from build123d import *

# Parameters (mm, degrees)
EXTRUDE_1_DEPTH             = 3
HOLE_WIZARD_M3_1_AT_2_COUNT = 2
HOLE_WIZARD_M3_1_AT_2_PITCH = 89
HOLE_WIZARD_M3_1_AT_3_COUNT = 2
HOLE_WIZARD_M3_1_AT_3_PITCH = 139.767316539
HOLE_WIZARD_M3_1_AT_4_COUNT = 2
HOLE_WIZARD_M3_1_AT_4_PITCH = 158.615198724
HOLE_WIZARD_M3_1_AT_5_COUNT = 2
HOLE_WIZARD_M3_1_AT_5_PITCH = 105.5
FILLET_1_R                  = 3
FILLET_2_R                  = 3
CUT_EXTRUDE_1_DEPTH         = 1.2
SKETCH_5_W                  = 15
SKETCH_5_H                  = 88
CUT_EXTRUDE_2_DEPTH         = 0.8
FILLET_5_R                  = 3
FILLET_6_R                  = 5
FILLET_7_R                  = 3
SKETCH_6_W                  = 1
SKETCH_6_H                  = 16
SKETCH_6_H_2                = 12
SKETCH_6_W_2                = 12
SKETCH_6_H_3                = 1
EXTRUDE_2_DEPTH             = 1
FILLET_8_R                  = 3
CHAMFER_1_SIZE              = 1
EXTRUDE_4_DEPTH             = 1.2
CUT_EXTRUDE_3_DEPTH         = 10
CUT_EXTRUDE_5_DEPTH         = 1.5
CUT_EXTRUDE_6_DEPTH         = 0.4
FILLET_9_R                  = 2
FILLET_10_R                 = 4


with BuildPart() as part:
    # 草图1 → 凸台-拉伸1 (new body)
    with BuildSketch(Plane.XY):
        Polygon((15, 96), (15, 72), (0, 72), (0, 10), (20, 0), (145, 0), (145, 96), align=None)
    extrude(amount=EXTRUDE_1_DEPTH)

    # 草图2 → M3 平头机械螺钉的锥形沉头孔1 (revolve, cut)
    with BuildSketch(Plane(origin=(141.5, 92.5, 3), x_dir=(0, -1, 0), z_dir=(1, 0, 0))):
        Polygon((0, 0), (0, 3), (1.7, 3), (1.7, 1.45), (3.15, 0), align=None)
    hole_wizard_m3_1 = revolve(axis=Axis((141.5, 92.5, 9.35), (0, 0, -1)), mode=Mode.SUBTRACT)

    # M3 平头机械螺钉的锥形沉头孔1 at 2: M3 平头机械螺钉的锥形沉头孔1 ×2
    with Locations(*[(0, -i * HOLE_WIZARD_M3_1_AT_2_PITCH, 0) for i in range(1, HOLE_WIZARD_M3_1_AT_2_COUNT)]):
        add(hole_wizard_m3_1, mode=Mode.SUBTRACT)

    # M3 平头机械螺钉的锥形沉头孔1 at 3: M3 平头机械螺钉的锥形沉头孔1 ×2
    with Locations(*[Vector(-0.9837779203696774, -0.1793906446644101, 0) * (i * HOLE_WIZARD_M3_1_AT_3_PITCH) for i in range(1, HOLE_WIZARD_M3_1_AT_3_COUNT)]):
        add(hole_wizard_m3_1, mode=Mode.SUBTRACT)

    # M3 平头机械螺钉的锥形沉头孔1 at 4: M3 平头机械螺钉的锥形沉头孔1 ×2
    with Locations(*[Vector(-0.8668778345720617, -0.4985206313961874, 0) * (i * HOLE_WIZARD_M3_1_AT_4_PITCH) for i in range(1, HOLE_WIZARD_M3_1_AT_4_COUNT)]):
        add(hole_wizard_m3_1, mode=Mode.SUBTRACT)

    # M3 平头机械螺钉的锥形沉头孔1 at 5: M3 平头机械螺钉的锥形沉头孔1 ×2
    with Locations(*[(-i * HOLE_WIZARD_M3_1_AT_5_PITCH, 0, 0) for i in range(1, HOLE_WIZARD_M3_1_AT_5_COUNT)]):
        add(hole_wizard_m3_1, mode=Mode.SUBTRACT)

    # 圆角1
    fillet_1_edges = [part.edges().sort_by_distance(p)[0] for p in [
        (145, 0, 1.5),
        (145, 96, 1.5),
    ]]
    fillet(fillet_1_edges, radius=FILLET_1_R)

    # 圆角2
    fillet_2_edges = [part.edges().sort_by_distance(p)[0] for p in [
        (20, 0, 1.5),
        (0, 10, 1.5),
        (0, 72, 1.5),
        (15, 96, 1.5),
    ]]
    fillet(fillet_2_edges, radius=FILLET_2_R)

    # 草图4 → 切除-拉伸1 (cut)
    with BuildSketch(Plane(origin=(0, 0, 0), x_dir=(-1, 0, 0), z_dir=(0, 0, -1))):
        Polygon((-133.585786438, 92), (-141, 84.585786438), (-141, 12.121320344), (-132.878679656, 4), (-22.062305899, 4), (-13, 8.531152949), (-13, 24), (-4, 27), (-4, 50.47410222), (-19.5, 68.946282906), (-19.5, 91), (-27.171572875, 91), (-32.171572875, 86), (-39.828427125, 86), (-45.828427125, 92), align=None)
    extrude(amount=-CUT_EXTRUDE_1_DEPTH, mode=Mode.SUBTRACT)

    # 草图5 → 切除-拉伸2 (cut)
    with BuildSketch(Plane(origin=(0, 0, 1.2), x_dir=(-1, 0, 0), z_dir=(0, 0, -1))):
        with Locations((-85.5, 48)):
            Rectangle(SKETCH_5_W, SKETCH_5_H)
    extrude(amount=-CUT_EXTRUDE_2_DEPTH, mode=Mode.SUBTRACT)

    # 圆角5
    fillet_5_edges = [part.edges().sort_by_distance(p)[0] for p in [
        (13, 8.531152949, 0.6),
        (22.062305899, 4, 0.6),
        (132.878679656, 4, 0.6),
        (141, 12.121320344, 0.6),
        (141, 84.585786438, 0.6),
        (133.585786438, 92, 0.6),
        (4, 50.47410222, 0.6),
        (4, 27, 0.6),
        (45.828427125, 92, 0.6),
        (27.171572875, 91, 0.6),
        (19.5, 91, 0.6),
    ]]
    fillet(fillet_5_edges, radius=FILLET_5_R)

    # 圆角6
    fillet_6_edges = [part.edges().sort_by_distance(p)[0] for p in [
        (39.828427125, 86, 0.6),
        (32.171572875, 86, 0.6),
        (19.5, 68.946282906, 0.6),
        (13, 24, 0.6),
    ]]
    fillet(fillet_6_edges, radius=FILLET_6_R)

    # 圆角7
    fillet_7_edges = [part.edges().sort_by_distance(p)[0] for p in [
        (78, 4, 1.6),
        (93, 4, 1.6),
        (78, 92, 1.6),
        (93, 92, 1.6),
    ]]
    fillet(fillet_7_edges, radius=FILLET_7_R)

    # 草图6 → 凸台-拉伸2 (add)
    with BuildSketch(Plane(origin=(0, 0, 0), x_dir=(-1, 0, 0), z_dir=(0, 0, -1))):
        with Locations((-141.5, 48)):
            Rectangle(SKETCH_6_W, SKETCH_6_H)
        with Locations((-3.5, 40)):
            Rectangle(SKETCH_6_W, SKETCH_6_H_2)
        with Locations((-76, 3.5)):
            Rectangle(SKETCH_6_W_2, SKETCH_6_H_3)
        with Locations((-76, 92.5)):
            Rectangle(SKETCH_6_W_2, SKETCH_6_H_3)
    extrude(amount=EXTRUDE_2_DEPTH)

    # 圆角8
    fillet_8_edges = [part.edges().sort_by_distance(p)[0] for p in [
        (15, 72, 1.5),
    ]]
    fillet(fillet_8_edges, radius=FILLET_8_R)

    # 倒角1
    chamfer_1_edges = [part.edges().sort_by_distance(p)[0] for p in [
        (3.5, 46, -1),
        (3.5, 34, -1),
        (70, 3.5, -1),
        (82, 3.5, -1),
        (141.5, 56, -1),
        (141.5, 40, -1),
        (82, 92.5, -1),
        (70, 92.5, -1),
    ]]
    chamfer(chamfer_1_edges, length=CHAMFER_1_SIZE - 0.0001)  # a hair under: the kernel refuses the full size

    # 草图9 → 凸台-拉伸4 (add)
    with BuildSketch(Plane(origin=(0, 0, 1.2), x_dir=(-1, 0, 0), z_dir=(0, 0, -1))):
        with BuildLine():
            Line((-95, 92), (-95, 34))
            Line((-95, 34), (-141, 34))
            Line((-141, 34), (-141, 83.343145751))
            ThreePointArc((-141, 83.343145751), (-140.771638598, 84.491196048), (-140.121320344, 85.464466094))
            Line((-140.121320344, 85.464466094), (-134.464466094, 91.121320344))
            ThreePointArc((-134.464466094, 91.121320344), (-133.491196048, 91.771638598), (-132.343145751, 92))
            Line((-132.343145751, 92), (-95, 92))
        make_face()
    extrude(amount=EXTRUDE_4_DEPTH)

    # 草图7 → 切除-拉伸3 (cut)
    with BuildSketch(Plane.XY.offset(3)):
        with BuildLine():
            Line((100, 86), (134, 86))
            ThreePointArc((134, 86), (134.707106781, 85.707106781), (135, 85))
            Line((135, 85), (135, 42))
            ThreePointArc((135, 42), (134.707106781, 41.292893219), (134, 41))
            Line((134, 41), (100, 41))
            ThreePointArc((100, 41), (99.292893219, 41.292893219), (99, 42))
            Line((99, 42), (99, 85))
            ThreePointArc((99, 85), (99.292893219, 85.707106781), (100, 86))
        make_face()
    extrude(amount=-CUT_EXTRUDE_3_DEPTH, mode=Mode.SUBTRACT)

    # 草图10 → 切除-拉伸5 (cut)
    with BuildSketch(Plane(origin=(0, 0, 0), x_dir=(-1, 0, 0), z_dir=(0, 0, -1))):
        with BuildLine():
            Line((-135, 89), (-99, 89))
            ThreePointArc((-99, 89), (-96.878679656, 88.121320344), (-96, 86))
            Line((-96, 86), (-96, 41))
            ThreePointArc((-96, 41), (-96.878679656, 38.878679656), (-99, 38))
            Line((-99, 38), (-135, 38))
            ThreePointArc((-135, 38), (-137.121320344, 38.878679656), (-138, 41))
            Line((-138, 41), (-138, 86))
            ThreePointArc((-138, 86), (-137.121320344, 88.121320344), (-135, 89))
        make_face()
    extrude(amount=-CUT_EXTRUDE_5_DEPTH, mode=Mode.SUBTRACT)

    # 草图12 → 切除-拉伸6 (cut)
    with BuildSketch(Plane(origin=(0, 0, 1.5), x_dir=(-1, 0, 0), z_dir=(0, 0, -1))):
        with BuildLine():
            Line((-135, 38), (-99, 38))
            ThreePointArc((-99, 38), (-96.878679656, 38.878679656), (-96, 41))
            Line((-96, 41), (-96, 86))
            ThreePointArc((-96, 86), (-96.878679656, 88.121320344), (-99, 89))
            Line((-99, 89), (-135, 89))
            ThreePointArc((-135, 89), (-137.121320344, 88.121320344), (-138, 86))
            Line((-138, 86), (-138, 41))
            ThreePointArc((-138, 41), (-137.121320344, 38.878679656), (-135, 38))
        make_face()
        with BuildLine():
            Line((-135, 39.5), (-99, 39.5))
            ThreePointArc((-99, 39.5), (-97.939339828, 39.939339828), (-97.5, 41))
            Line((-97.5, 41), (-97.5, 86))
            ThreePointArc((-97.5, 86), (-97.939339828, 87.060660172), (-99, 87.5))
            Line((-99, 87.5), (-135, 87.5))
            ThreePointArc((-135, 87.5), (-136.060660172, 87.060660172), (-136.5, 86))
            Line((-136.5, 86), (-136.5, 41))
            ThreePointArc((-136.5, 41), (-136.060660172, 39.939339828), (-135, 39.5))
        make_face(mode=Mode.SUBTRACT)
    extrude(amount=-CUT_EXTRUDE_6_DEPTH, mode=Mode.SUBTRACT)

    # 圆角9
    fillet_9_edges = [part.edges().sort_by_distance(p)[0] for p in [
        (141, 34, 0.6),
        (95, 92, 0.6),
    ]]
    fillet(fillet_9_edges, radius=FILLET_9_R)

    # 圆角10
    fillet_10_edges = [part.edges().sort_by_distance(p)[0] for p in [
        (95, 34, 0.6),
    ]]
    fillet(fillet_10_edges, radius=FILLET_10_R)


solid = part.part
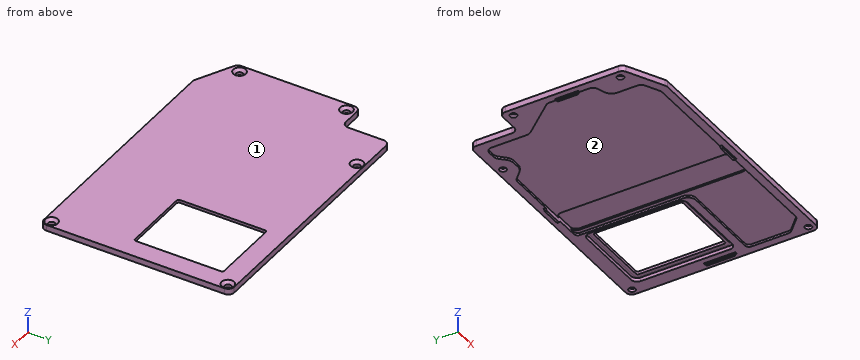
Part model, mm, in its own coordinate system. Face numbers are marked on the shaded views. Coordinates: 2 decimals unless noted, no trailing zeros. Order: outer loops, then holes, each group sorted by start corner. A loop starts at its lowest first (then second) coordinate and runs counter-clockwise, first axis right, second up. Notation, with made-up numbers: M 5,-17 L 32,-17 A31 cw 32,13 Z; hole C -18,84 d3. An arc over 180 degrees is marked long. Use a Markdown table: item, result.
(1) Cut at C-C on x = 103. Write the cut outline in (y, z).
A:
| item | result |
|---|---|
| outline | M 0,0 L 4,0 L 4,1.2 L 34,1.2 L 34,0 L 38,0 L 38,1.9 L 39.5,1.9 L 39.5,1.5 L 41,1.5 L 41,3 L 0,3 Z; M 86,1.5 L 87.5,1.5 L 87.5,1.9 L 89,1.9 L 89,0 L 96,0 L 96,3 L 86,3 Z |
(2) Flat gauge pins, fed straight in: pin 1 (1.5 mm diameter, centred on y = 85.5, z = 1.5, fed in from -X); pin 2 (2 mm diameter, centred on x = 141.5, y = 92.5, fed in from -Z); pin 3 (4.5 mm diameter, centred on x = 4, y = 13.43, fed in from -Z). Where does each tip first touch, or does it go through?
A:
| item | result |
|---|---|
| pin 1 | stops at x = 15 |
| pin 2 | passes through |
| pin 3 | stops at z = 0 |
(3) Cut at A-A on x = 36. Write the cut outline in (y, z), then the cut area to 3 significant figures.
A:
| item | result |
|---|---|
| outline | M 0,0 L 4,0 L 4,1.2 L 86,1.2 L 86,0 L 90.8,0 L 90.8,1.55 L 89.35,3 L 0,3 Z; M 94.2,0 L 96,0 L 96,3 L 95.65,3 L 94.2,1.55 Z |
| area | 177 mm^2 |
(4) Cut at B-B on x = 50.5. Write the cut outline in (y, z), then the cut area to 3 significant figures.
A:
| item | result |
|---|---|
| outline | M 0,0 L 4,0 L 4,1.2 L 92,1.2 L 92,0 L 96,0 L 96,3 L 0,3 Z |
| area | 182 mm^2 |
(5) Pull direction X, two halves, no side cores. Call the marked faces 1 and 2: released by +X, released by -X, zero draft, split by the parting line, or undercut.
A:
| item | result |
|---|---|
| face 1 | zero draft |
| face 2 | undercut |
(6) Probe L1, parallel to Y at x = 116.5, z = 0.9; L2, parallel to Y at x = 141.5, z = 0.6; L3, parallel to X at y = 92.5, z = 1.25. List the from-to ranges inside material, lowest first.
A:
| item | result |
|---|---|
| L1 | y = 0 to 4, 34 to 38, 89 to 96 |
| L2 | y = 0 to 1.8, 5.2 to 90.8, 94.2 to 96 |
| L3 | x = 15 to 34.3, 37.7 to 139.8, 143.2 to 145 |
